Verification items for the finished model (mm, model axes). A direction names the side the tool comes from. Round coordinates to 2 decimals unless told otherwise and drop trailing zeros. Order: outer loops, then holes, each group sorted by start corner. A loop starts at its lowest first (then second) coordinate and runs counter-clockwise, first axis right, second up. Notation, with made-up numbers: (16, -32) -> (43, -32) arc R26 ccw to (43, -18) -> close; hole circle Ø10 at (21.25, 50). An arc over 180 degrees is marked (long way). Return JSON: item names as keys, results as strings. Group by question number.
Item 1: Scan lines: probe 1 along Z at (x, y) = (-1.5, 0); probe 2 along Z at (x, y) = (-3.25, -2.25); probe 3 along Z at (x, y) = (-4.5, 5.5). Record each from-to range of solid material in increasing order. Write a range as from..to.
Item 2: Sectioned sample at D-D on y = 3.75. Record the cut outline in (x, z).
Item 3: Sectioned sample at B-B on x = -1. Record the cut outline in (y, z), plus the area to 3 significant figures.
Item 4: Access from +Z, -Z, +X, -X, +Y, -Y to the whole of each face (thin tool, end or side, straight path). Record for faces 5 (the flat face through (-3.5, 4.3, 15.6)), 6 (the flat face through (0, -6.75, 12)).
Item 5: Draft check along Y on faces 1 (the flat face through (-2, -2.5, 20.3)), 2 (the flat face through (-4, 0, 13.1)), 3 (the flat face through (5, 0, 12)), 4 (the cylindrical face through (0.07, -6.18, 0.6)). Enter one of: pulls with the +Y half, pulls with the -Y half, needs draft (parallel to the pull), parting line crosses it, or undercut.
Item 6: Depth check by flat-ended pin: pin 1 Ø8 at (y, z) = (0, 18.05) entering from -X; pin 2 Ø1 at (x, y) = (3, -5) entering from +Z. Enter the tip coordinate at first touch or a pass-through.
Item 7: Sectioned sample at C-C on y = -2. Record the cut outline in (x, z), plus the area to 3 significant figures.
Item 8: Sectioned sample at A-A on z = 5. Record the cut outline in (x, y), plus the area to 3 significant figures.
```python
from build123d import *

# Parameters (mm, degrees)
F0_W     = 10
F0_H     = 13.5
F1_DEPTH = 25
F2_R     = 3
F3_DEPTH = 3
F4_DEPTH = 25
F5_R     = 2


with BuildPart() as f1:
    # F0 (on Top) → F1 (new body)
    with BuildSketch(Plane.XY):
        Rectangle(F0_W, F0_H)
    extrude(amount=F1_DEPTH)

    # F2 (on face) → F3 (cut)
    with BuildSketch(Plane(origin=(-5, 0, 0), x_dir=(0, -1, 0), z_dir=(-1, 0, 0))):
        Polygon((2.857884, 23), (-2.857884, 23), (-5.715768, 18.05), (-2.857884, 13.1), (2.857884, 13.1), (5.715768, 18.05), align=None)
        with Locations((0, 18.05)):
            Circle(F2_R, mode=Mode.SUBTRACT)
    extrude(amount=-F3_DEPTH, mode=Mode.SUBTRACT)

    # F2 (on face) → F4 (cut)
    with BuildSketch(Plane(origin=(-5, 0, 0), x_dir=(0, -1, 0), z_dir=(-1, 0, 0))):
        with Locations((0, 5)):
            Circle(F2_R)
        with Locations((0, 18.05)):
            Circle(F2_R)
    extrude(amount=-F4_DEPTH, mode=Mode.SUBTRACT)

    # F5
    f5_edges = [f1.edges().sort_by_distance(p)[0] for p in [
        (0, -6.75, 25),
        (0, 6.75, 25),
        (0, -6.75, 0),
        (0, 6.75, 0),
    ]]
    fillet(f5_edges, radius=F5_R)


solid = f1.part
```
Recorded:
{
 "1": {"probe 1": "0..2, 8..15.05, 21.05..25", "probe 2": "0..3.02, 6.98..13.1, 23..25", "probe 3": "0.15..17.68, 18.42..24.85"},
 "2": {"outline": "(-5, 0) -> (5, 0) -> (5, 25) -> (-5, 25) -> (-5, 21.45) -> (-2, 21.45) -> (-2, 14.65) -> (-5, 14.65) -> close"},
 "3": {"outline": "(-6.75, 2) arc R2 ccw to (-4.75, 0) -> (4.75, 0) arc R2 ccw to (6.75, 2) -> (6.75, 23) arc R2 ccw to (4.75, 25) -> (-4.75, 25) arc R2 ccw to (-6.75, 23) -> close; hole circle Ø6 at (0, 5); hole circle Ø6 at (0, 18.05)", "area": "278 mm²"},
 "4": {"face 5": "-X", "face 6": "+Z, -Z, +X, -X, -Y"},
 "5": {"face 1": "undercut", "face 2": "undercut", "face 3": "needs draft", "face 4": "pulls with the -Y half"},
 "6": {"pin 1": "x = -2", "pin 2": "z = 25"},
 "7": {"outline": "(-5, 0) -> (5, 0) -> (5, 2.76) -> (-5, 2.76) -> close; (-5, 7.24) -> (5, 7.24) -> (5, 15.81) -> (-2, 15.81) -> (-2, 13.1) -> (-5, 13.1) -> close; (-5, 23) -> (-2, 23) -> (-2, 20.29) -> (5, 20.29) -> (5, 25) -> (-5, 25) -> close", "area": "144 mm²"},
 "8": {"outline": "(-5, -6.75) -> (5, -6.75) -> (5, -3) -> (-5, -3) -> close; (-5, 3) -> (5, 3) -> (5, 6.75) -> (-5, 6.75) -> close", "area": "75.0 mm²"}
}
